The model under review builds one solid part; all positions refer to its coordinate system, in mm. Round coordinates to 2 decimals unless told otherwise and drop trailing zeros. Write each loop counter-clockwise with the first axis right and the second up, starting at its lowest first coordinate (ties: lowest second). Pieces come first, ordered by that corner, then holes. Notation, with made-up numbers: (79, -10.75) - (107, -10.75) arc R20 cw to (107, -5.75) - close; hole circle Ø6 at (87, -30.75). An arc over 180 degrees is marked (long way). Use one line per item in the form item = value.
from build123d import *


with BuildPart() as part:
    # Skizze1 → Rotation1 (revolve)
    with BuildSketch(Plane(origin=(0, 0, 0), x_dir=(0, 0, -1), z_dir=(1, 0, 0)), mode=Mode.PRIVATE) as rotation1_sk:
        Polygon((-7.315845432, 0), (-7.315845432, 5), (-5.315845432, 5), (-5.315845432, 4.292030432), (-4.315845432, 4.292030432), (-4.315845432, 5), (46.684154568, 5), (46.684154568, 4.292030432), (47.684154568, 4.292030432), (47.684154568, 5), (50.684154568, 5), (50.684154568, 4.255858279), (51.684154568, 4.255858279), (51.684154568, 5), (79.684154568, 5), (79.684154568, 4.292030432), (80.684154568, 4.292030432), (80.684154568, 5), (82.684154568, 5), (82.684154568, 0), align=None)
    revolve(rotation1_sk.sketch.rotate(Axis((0, 0, 7.315845432), (0, 0, -1)), 90), axis=Axis((0, 0, 7.315845432), (0, 0, -1)))


solid = part.part
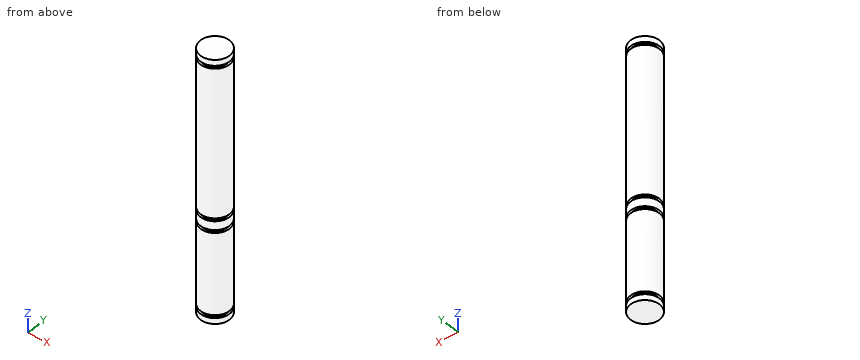
(1) To check wall thickness, follow L1, parallel to Z at x = 2.75, y = -3.5; L2, parallel to Y at x = 0.25, z = -2. State the ranges of each line that lie inside material, in increasing order.
Geometry results:
L1 = -82.68 to -80.68, -79.68 to -51.68, -50.68 to -47.68, -46.68 to 4.32, 5.32 to 7.32
L2 = -4.99 to 4.99
(2) Add section A-A on z = -74. Write out the cut boundary in (x, y), then the cut area to 3 significant figures.
Geometry results:
outline = circle Ø10 at (0, 0)
area = 78.5 mm2
(3) Insertion check: P1, Ø1.5, axis at y = -4, z = -22.5, coming from the +X side; P2, Ø1, axis at y = 2.5, z = -26.5, coming from the +X side; P3, Ø1.5, axis at x = 4, z = -39, coming from the -Y side. Each pin has a flat end and moves straight along its axis. Give the tip position at first contact, or say it passes through.
Geometry results:
P1 = 3.8
P2 = 4.58
P3 = -3.8
